```python
from build123d import *

# Parameters (mm, degrees)
F0_R     = 19.05
F1_DEPTH = 2.5
F2_R     = 6.45
F2_R_2   = 6.35
F3_DEPTH = 0.5
F4_DEPTH = 0.5


with BuildPart() as f1:
    # F0 (on Top) → F1 (new body)
    with BuildSketch(Plane.XY):
        Circle(F0_R)
    extrude(amount=F1_DEPTH)

    # F2 (on face) → F3 (cut)
    with BuildSketch(Plane.XY.offset(2.5)):
        Circle(F2_R)
        Circle(F2_R_2, mode=Mode.SUBTRACT)
    extrude(amount=-F3_DEPTH, mode=Mode.SUBTRACT)

    # F2 (on face) → F4 (cut)
    with BuildSketch(Plane.XY.offset(2.5)):
        Circle(F2_R)
        Circle(F2_R_2, mode=Mode.SUBTRACT)
    extrude(amount=-F4_DEPTH, mode=Mode.SUBTRACT)

    # F5 (on Front) → F6 (revolve)
    with BuildSketch(Plane.XZ):
        with BuildLine():
            Line((0, -2.375183), (0, 0))
            Line((0, 0), (-19.05, 0))
            ThreePointArc((-19.05, 0), (-16.407129, -1.284926), (-13.678185, -2.375183))
            Line((-13.678185, -2.375183), (0, -2.375183))
        make_face()
    revolve(axis=Axis((0, 0, -1.187592), (0, 0, -1)))


solid = f1.part
```
CAD build for the part. Positions are in the model's coordinates, mm. Coordinates: 2 decimals unless noted, no trailing zeros. Write each loop counter-clockwise with the first axis right and the second up, starting at its lowest first coordinate (ties: lowest second). Pieces come first, ordered by that corner, then holes.
(1) Two-plate mould, pull along X, no slides. Class faces 1 (the face through (-15.12, -11.59, 1.23)), 2 (the face through (0, 0, 2.5)): +X half, -X half, draft (parallel to the pull), parting line (faces both ways), or undercut.
(2) Drill centre lines: probe 1 along X at (y, z) = (0.5, 1.85); probe 2 along X at (y, z) = (11.5, 0.75); probe 3 along Y at (x, z) = (2.5, -0.55). Where is each one in solid material? Low to high.
(3) Cut at A-A, the plane z = 1.25. List the corners of the cut face in (x, y).
(4) Flat gauge pins, fed straight in: pin 1 (1.5 mm diameter, centred on x = 9, z = 1.5, fed in from +Y); pin 2 (1.5 mm diameter, centred on y = -9.5, z = 0.5, fed in from +X); pin 3 (5 mm diameter, centred on x = 14, y = -3.5, fed in from -Z). Where does each tip first touch, or does it go through?
Geometry says:
1. face 1: parting line
1. face 2: draft
2. probe 1: x = -19.04 to 19.04
2. probe 2: x = -15.19 to 15.19
2. probe 3: y = -17.8 to 17.8
3. outline: circle Ø38.1 at (0, 0)
4. pin 1: stops at y = 17.17
4. pin 2: stops at x = 16.92
4. pin 3: stops at z = -2.38
